Design review of the part built by this model. Coordinates are the model's own, in mm. Face numbers are marked on the shaded views. A direction names the side the tool comes from. Give positions to 0.01 mm unless a question says otherwise; leave off trailing zeros. Loops run counter-clockwise (first coordinate to the right, second up) from the corner with the lowest first, then second, coordinate; pieces in that order, holes last.
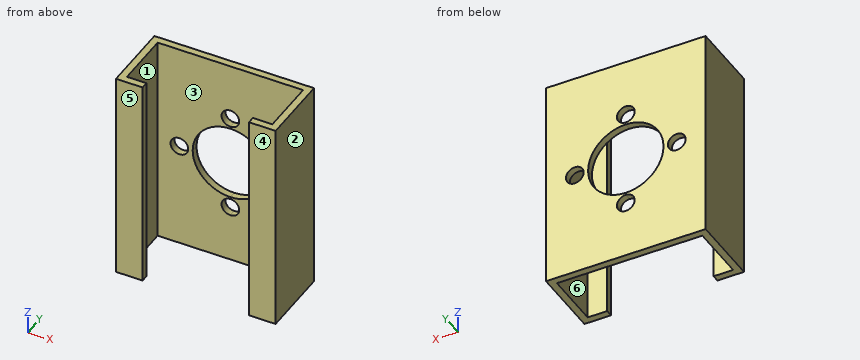
from build123d import *

# Parameters (mm, degrees)
F1_DEPTH = 48
F3_DEPTH = 25
F4_DEPTH = 25
F5_DEPTH = 25


with BuildPart() as f1:
    # F0 (on Top) → F1 (new body)
    with BuildSketch(Plane.XY):
        Polygon((12, -8), (18, -8), (18, 8), (-18, 8), (-18, -8), (-12, -8), (-12, -6.4), (-16.4, -6.4), (-16.4, 6.4), (16.4, 6.4), (16.4, -6.4), (12, -6.4), align=None)
    extrude(amount=F1_DEPTH)

    # F2 (on face) → F3 (cut)
    with BuildSketch(Plane.XZ.offset(-6.4)):
        with BuildLine():
            Line((0, 24), (0, 32.5))
            ThreePointArc((0, 32.5), (-6.0104076401, 30.0104076401), (-8.5, 24))
            Line((-8.5, 24), (0, 24))
        make_face()
        with BuildLine():
            ThreePointArc((8.5, 24), (6.0104076401, 30.0104076401), (0, 32.5))
            Line((0, 32.5), (0, 24))
            Line((0, 24), (8.5, 24))
        make_face()
        with BuildLine():
            Line((0, 15.5), (0, 24))
            Line((0, 24), (-8.5, 24))
            ThreePointArc((-8.5, 24), (-6.0104076401, 17.9895923599), (0, 15.5))
        make_face()
        with BuildLine():
            Line((8.5, 24), (0, 24))
            Line((0, 24), (0, 15.5))
            ThreePointArc((0, 15.5), (6.0104076401, 17.9895923599), (8.5, 24))
        make_face()
    extrude(amount=-F3_DEPTH, mode=Mode.SUBTRACT)

    # F2 (on face) → F4 (cut)
    with BuildSketch(Plane.XZ.offset(-6.4)):
        with BuildLine():
            Line((0, 15), (0, 11))
            ThreePointArc((0, 11), (1.4142135624, 11.5857864376), (2, 13))
            ThreePointArc((2, 13), (1.4142135624, 14.4142135624), (0, 15))
        make_face()
        with BuildLine():
            ThreePointArc((0, 15), (-2, 13), (0, 11))
            Line((0, 11), (0, 15))
        make_face()
        with BuildLine():
            Line((0, 33), (0, 37))
            ThreePointArc((0, 37), (-2, 35), (0, 33))
        make_face()
        with BuildLine():
            ThreePointArc((2, 35), (1.4142135624, 36.4142135624), (0, 37))
            Line((0, 37), (0, 33))
            ThreePointArc((0, 33), (1.4142135624, 33.5857864376), (2, 35))
        make_face()
    extrude(amount=-F4_DEPTH, mode=Mode.SUBTRACT)

    # F2 (on face) → F5 (cut)
    with BuildSketch(Plane.XZ.offset(-6.4)):
        with BuildLine():
            Line((-9.5, 24), (-13.5, 24))
            ThreePointArc((-13.5, 24), (-11.5, 22), (-9.5, 24))
        make_face()
        with BuildLine():
            ThreePointArc((-9.5, 24), (-11.5, 26), (-13.5, 24))
            Line((-13.5, 24), (-9.5, 24))
        make_face()
        with BuildLine():
            Line((9.5, 24), (13.5, 24))
            ThreePointArc((13.5, 24), (11.5, 26), (9.5, 24))
        make_face()
        with BuildLine():
            ThreePointArc((9.5, 24), (11.5, 22), (13.5, 24))
            Line((13.5, 24), (9.5, 24))
        make_face()
    extrude(amount=-F5_DEPTH, mode=Mode.SUBTRACT)


solid = f1.part
Q1. Take a section at C-C (z = 43.5). Give the boundary of the cut face in (x, y), plus the area to 3 significant figures.
Results:
outline: (-18, -8) - (-12, -8) - (-12, -6.4) - (-16.4, -6.4) - (-16.4, 6.4) - (16.4, 6.4) - (16.4, -6.4) - (12, -6.4) - (12, -8) - (18, -8) - (18, 8) - (-18, 8) - close
area: 118 mm2
Q2. Tool access review of the marked faces 5 and 6: name each direction out of +Z, -Z, +X, -X, +Y, -Y from which nothing blocks a thin tool from reaching the whole face with its end or side.
Results:
face 5: +Z, -Z, +X, -X, -Y
face 6: +Z, -Z
Q3. Insertion check: pin 1 (2.5 mm diameter, centred on x = -11.5, z = 24, fed in from +Y); pin 2 (1 mm diameter, centred on x = 10, z = 30.5, fed in from -Y). Each pin has a flat end and moves straight along its axis. Give the tip position at first contact, or say it passes through.
Results:
pin 1: stops at y = -6.4
pin 2: stops at y = 6.4
Q4. Draft analysis for pull direction X (two halves, no side actions). For the marked faces 1, 2, 3 and 4, state which applies: pulls with the +X half, pulls with the -X half, needs draft (parallel to the pull), parting line crosses it, or undercut.
Results:
face 1: undercut
face 2: pulls with the +X half
face 3: undercut
face 4: needs draft
Q5. Take a section at B-B (y = 0). Give the boundary of the cut face in (x, z), plus the area to 3 significant figures.
Results:
outline: (-18, 0) - (-16.4, 0) - (-16.4, 48) - (-18, 48) - close; (16.4, 0) - (18, 0) - (18, 48) - (16.4, 48) - close
area: 154 mm2
Q6. Take a section at A-A (x = -11.5). Give the boundary of the cut face in (y, z), plus the area to 3 significant figures.
Results:
outline: (6.4, 0) - (8, 0) - (8, 22) - (6.4, 22) - close; (6.4, 26) - (8, 26) - (8, 48) - (6.4, 48) - close
area: 70.4 mm2
Q7. Wall thickness on line 1 (X direction, y = -1.5, z = 44); line 2 (Z direction, x = -11.5, y = 7.05); line 3 (Y direction, x = 2.5, z = 4): over which ranges is each line inside the solid? List them lowest first.
Results:
line 1: x = -18 to -16.4, 16.4 to 18
line 2: z = 0 to 22, 26 to 48
line 3: y = 6.4 to 8
Q8. Take a section at D-D (x = -1.5). Give the boundary of the cut face in (y, z).
Results:
outline: (6.4, 0) - (8, 0) - (8, 11.68) - (6.4, 11.68) - close; (6.4, 14.32) - (8, 14.32) - (8, 15.63) - (6.4, 15.63) - close; (6.4, 32.37) - (8, 32.37) - (8, 33.68) - (6.4, 33.68) - close; (6.4, 36.32) - (8, 36.32) - (8, 48) - (6.4, 48) - close
